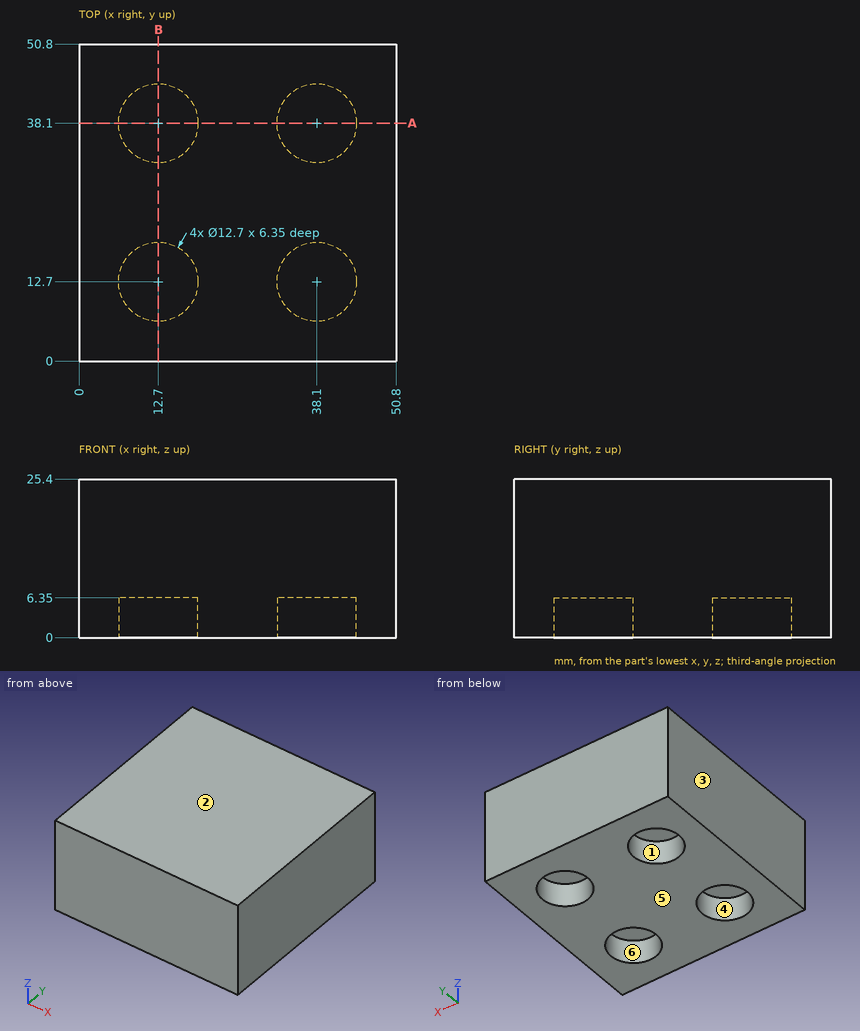
Geometry: see drawing. Coordinates: mm, zero at the bounding-box minimum. A direction names the side the tool comes from. Coordinates: 2 decimals unless noted, no trailing zeros. Order: outer loops, then holes, each group sorted by start corner. A loop starts at its lowest first (then second) coordinate and runs counter-clockwise, first axis right, second up. Notation, with made-up numbers: M -18.5,53.5 L 16.5,53.5 A23 ccw 16.5,90.5 Z; hole C 59.25,24.5 d10. An arc over 180 degrees is marked long. Answer in a Markdown table with one row per item. Add a question column.
Q1. Contact query for a flat-ended pin moving along its axis: P1, Ø4, axis at x = 38.5, y = 13, coming from the -Z side. Output: stop coordinate, or through.
Q2. Section query A-A on y = 38.1. Return the cut outline in (x, z).
Q3. Reachability of the marked faces 5 and 6 from +Z, -Z, +X, -X, +Y, -Y: full face, straight path, thin tool, end or side. Return the list, or none.
Q4. Mould query, pull axis X, two halves, no side actions, for the marked faces 1, 2, 3 and 4. Classes: released by +X, released by -X, zero draft, split by the parting line, or undercut.
Q5. Line query: L1, parallel to X at y = 12.7, z = 2.75; L2, parallel to X at y = 16, z = 1.75. Output: solid intervals per line, ascending.
Completed:
| question | item | result |
|---|---|---|
| 1 | P1 | stops at z = 6.35 |
| 2 | outline | M 0,0 L 6.35,0 L 6.35,6.35 L 19.05,6.35 L 19.05,0 L 31.75,0 L 31.75,6.35 L 44.45,6.35 L 44.45,0 L 50.8,0 L 50.8,25.4 L 0,25.4 Z |
| 3 | face 5 | -Z, +X, -X, +Y, -Y |
| 3 | face 6 | -Z |
| 4 | face 1 | undercut |
| 4 | face 2 | zero draft |
| 4 | face 3 | released by -X |
| 4 | face 4 | undercut |
| 5 | L1 | x = 0 to 6.35, 19.05 to 31.75, 44.45 to 50.8 |
| 5 | L2 | x = 0 to 7.27, 18.13 to 32.67, 43.53 to 50.8 |
